```python
from build123d import *

# Parameters (mm, degrees)
F0_W     = 130
F0_H     = 50
F1_DEPTH = 25
F2_T     = -2.5
F3_R     = 1.75
F4_DEPTH = 1.5
F5_W     = 10
F5_H     = 2.5
F6_DEPTH = 2.5


with BuildPart() as f1:
    # F0 (on Top) → F1 (new body)
    with BuildSketch(Plane.XY):
        with Locations((65, 0)):
            Rectangle(F0_W, F0_H)
    extrude(amount=F1_DEPTH)

    # F2
    f2_openings = [f1.faces().sort_by_distance(p)[0] for p in [
        (65, 0, 25),
    ]]
    offset(amount=F2_T, openings=f2_openings)

    # F3 (on face) → F4 (join)
    with BuildSketch(Plane(origin=(0, 0, 0), x_dir=(1, 0, 0), z_dir=(0, 0, -1))):
        with Locations((7.5, 0)):
            Circle(F3_R)
    extrude(amount=F4_DEPTH)

    # F5 (on face) → F6 (cut, through all)
    with BuildSketch(Plane(origin=(0, 0, 0), x_dir=(1, 0, 0), z_dir=(0, 0, -1))):
        with Locations((55, -1.25)):
            Rectangle(F5_W, F5_H)
        with Locations((78, -1.25)):
            Rectangle(F5_W, F5_H)
    extrude(amount=-F6_DEPTH, mode=Mode.SUBTRACT)


solid = f1.part
```
The model under review builds one solid part; all positions refer to its coordinate system, in mm. A direction names the side the tool comes from. Round coordinates to 2 decimals unless told otherwise and drop trailing zeros. Write each loop counter-clockwise with the first axis right and the second up, starting at its lowest first coordinate (ties: lowest second). Pieces come first, ordered by that corner, then holes.
(1) Wall thickness on L1, parallel to Y at x = 87, z = 7.5; L2, parallel to X at y = -12.5, z = 18; L3, parallel to Z at x = 120.5, y = 21: over which ranges is each line inside the solid? List them lowest first.
(2) Machinability: for faces 1 (the flat face through (64, 0, 2.5)), 2 (the flat face through (64, 25, 12)), 3 (the flat face through (60, 1, 1)), 4 (the cylindrical face through (9.169, -0.526, -0.74)), which of the approach directions +Z, -Z, +X, -X, +Y, -Y give a long, thin tool a straight path to every point of the face, cutting with its end or side? Answer none if there is none.
(3) Mouldability with a two-part tool opening along X and no side actions: class faces 5 (the flat face through (130, 0, 12)), 6 (the flat face through (55, 2.5, 1)), 7 (the flat face through (0, 0, 12)), 8 (the flat face through (64, 0, 0)) as +X half, -X half, draft (parallel to the pull), parting line (faces both ways), or undercut.
(4) We need section A-A on x = 54.5. Give the boundary of the cut face in (y, z), and give its area (3 significant figures).
(5) We need section B-B on y = -13. Give the boundary of the cut face in (x, z), and give its area (4 significant figures).
(6) We need section D-D on z = 6. Give the boundary of the cut face in (x, y).
(7) Insertion check: pin 1 (12 mm diameter, centred on x = 115.5, y = 0.5, fed in from -Z). The pin has a flat end and moves straight along its axis. Give the tip position at first contact, or say it passes through.
(8) We need section C-C on x = 88. Give the boundary of the cut face in (y, z).
Findings below:
1. L1: y = -25 to -22.5, 22.5 to 25
1. L2: x = 0 to 2.5, 127.5 to 130
1. L3: z = 0 to 2.5
2. face 1: +Z
2. face 2: +Z, -Z, +X, -X, +Y
2. face 3: +Z, -Z
2. face 4: -Z
3. face 5: +X half
3. face 6: undercut
3. face 7: -X half
3. face 8: draft
4. outline: (-25, 0) - (0, 0) - (0, 2.5) - (-22.5, 2.5) - (-22.5, 25) - (-25, 25) - close; (2.5, 0) - (25, 0) - (25, 25) - (22.5, 25) - (22.5, 2.5) - (2.5, 2.5) - close
4. area: 231 mm2
5. outline: (0, 0) - (130, 0) - (130, 25) - (127.5, 25) - (127.5, 2.5) - (2.5, 2.5) - (2.5, 25) - (0, 25) - close
5. area: 437.5 mm2
6. outline: (0, -25) - (130, -25) - (130, 25) - (0, 25) - close; hole (2.5, -22.5) - (127.5, -22.5) - (127.5, 22.5) - (2.5, 22.5) - close
7. pin 1: stops at z = 0
8. outline: (-25, 0) - (25, 0) - (25, 25) - (22.5, 25) - (22.5, 2.5) - (-22.5, 2.5) - (-22.5, 25) - (-25, 25) - close
